```python
from build123d import *

# Parameters (mm, degrees)
F2_R     = 1.5
F3_DEPTH = 12.5
F2_R_2   = 1.75
F4_DEPTH = 4.75
F5_R     = 1.875
F5_R_2   = 1.75
F6_DEPTH = 0.2
F7_R     = 1.875
F7_R_2   = 1.75
F8_DEPTH = 0.2


with BuildPart() as f1:
    # F0 (on Front) → F1 (revolve)
    with BuildSketch(Plane.XZ):
        with BuildLine():
            ThreePointArc((-4, 0), (0, -4), (4, 0))
            Line((4, 0), (-4, 0))
        make_face()
    revolve(axis=Axis((3.253754, 0, 0), (1, 0, 0)))

    # F2 (on Front) → F3 (cut, symmetric)
    with BuildSketch(Plane.XZ):
        Circle(F2_R)
    extrude(amount=F3_DEPTH, both=True, mode=Mode.SUBTRACT)

    # F2 (on Front) → F4 (join, symmetric)
    with BuildSketch(Plane.XZ):
        Circle(F2_R_2)
        Circle(F2_R, mode=Mode.SUBTRACT)
    extrude(amount=F4_DEPTH, both=True)

    # F5 (on face) → F6 (join)
    with BuildSketch(Plane.XZ.offset(4.75)):
        Circle(F5_R)
        Circle(F5_R_2, mode=Mode.SUBTRACT)
    extrude(amount=-F6_DEPTH)

    # F7 (on face) → F8 (join)
    with BuildSketch(Plane(origin=(0, 4.75, 0), x_dir=(-1, 0, 0), z_dir=(0, 1, 0))):
        Circle(F7_R)
        Circle(F7_R_2, mode=Mode.SUBTRACT)
    extrude(amount=-F8_DEPTH)


solid = f1.part
```
CAD build for the part. Positions are in the model's coordinates, mm. Give positions to 0.01 mm unless a question says otherwise; leave off trailing zeros. Order: outer loops, then holes, each group sorted by start corner. A loop starts at its lowest first (then second) coordinate and runs counter-clockwise, first axis right, second up.
(1) Saw through at C-C, the plane y = -1.5. Give the cut face in (x, z), then the cut area to 3 significant figures.
(2) Saw through at D-D, the plane y = 1.75. Give the cut face in (x, z), then the cut area to 3 significant figures.
(3) Drill centre lines: L1, parallel to Z at x = 0, y = 4.45; L2, parallel to Z at x = 0, y = -2.75. Where is each one in solid material? Low to high.
(4) Flat gauge pins, fed straight in: pin 1 (1.9 mm diameter, centred on x = -0.5, z = 0.5, fed in from +Y); pin 2 (4 mm diameter, centred on x = 2, y = -2, fed in from -Z); pin 3 (1.5 mm diameter, centred on y = 1.5, z = -2.5, fed in from -X); pin 4 (1.5 mm diameter, centred on y = -3.5, z = 0, fed in from +X). Where does each tip first touch, or does it go through?
(5) Saw through at B-B, the plane x = 0. Give the cut face in (y, z) (3 decimals).
(6) Saw through at A-A, the plane z = 0. Give the cut face in (x, y) (3 decimals).
Results found:
1. outline: circle Ø7.42 at (0, 0); hole circle Ø3 at (0, 0)
1. area: 36.1 mm2
2. outline: circle Ø7.19 at (0, 0); hole circle Ø3 at (0, 0)
2. area: 33.6 mm2
3. L1: z = -1.75 to -1.5, 1.5 to 1.75
3. L2: z = -2.9 to -1.5, 1.5 to 2.9
4. pin 1: stops at y = 4.75
4. pin 2: stops at z = -3.91
4. pin 3: stops at x = -3.36
4. pin 4: stops at x = 2.9
5. outline: (-4.75, -1.875) - (-4.55, -1.875) - (-4.55, -1.75) - (-3.597, -1.75) arc R4 ccw to (3.597, -1.75) - (4.55, -1.75) - (4.55, -1.875) - (4.75, -1.875) - (4.75, -1.5) - (-4.75, -1.5) - close; (-4.75, 1.5) - (4.75, 1.5) - (4.75, 1.875) - (4.55, 1.875) - (4.55, 1.75) - (3.597, 1.75) arc R4 ccw to (-3.597, 1.75) - (-4.55, 1.75) - (-4.55, 1.875) - (-4.75, 1.875) - close
6. outline: (-1.875, -4.75) - (-1.5, -4.75) - (-1.5, 4.75) - (-1.875, 4.75) - (-1.875, 4.55) - (-1.75, 4.55) - (-1.75, 3.597) arc R4 ccw to (-1.75, -3.597) - (-1.75, -4.55) - (-1.875, -4.55) - close; (1.5, -4.75) - (1.875, -4.75) - (1.875, -4.55) - (1.75, -4.55) - (1.75, -3.597) arc R4 ccw to (1.75, 3.597) - (1.75, 4.55) - (1.875, 4.55) - (1.875, 4.75) - (1.5, 4.75) - close
